```python
from build123d import *

# Parameters (mm, degrees)
CROQUIS1_W              = 128
CROQUIS1_H              = 98
SALIENTE_EXTRUIR1_DEPTH = 11.8
CROQUIS2_W              = 126
CROQUIS2_H              = 96
CORTAR_EXTRUIR1_DEPTH   = 11.3
SALIENTE_EXTRUIR2_DEPTH = 128
CROQUIS7_R              = 2.5
CORTAR_EXTRUIR2_DEPTH   = 22


with BuildPart() as part:
    # Croquis1 → Saliente-Extruir1 (new body)
    with BuildSketch(Plane.XY):
        with Locations((-9.684466696, -19.00455338)):
            Rectangle(CROQUIS1_W, CROQUIS1_H)
    extrude(amount=SALIENTE_EXTRUIR1_DEPTH)

    # Croquis2 → Cortar-Extruir1 (cut)
    with BuildSketch(Plane.XY.offset(11.8)):
        with Locations((-9.684466696, -19.00455338)):
            Rectangle(CROQUIS2_W, CROQUIS2_H)
    extrude(amount=-CORTAR_EXTRUIR1_DEPTH, mode=Mode.SUBTRACT)

    # Croquis5 → Saliente-Extruir2 (add)
    with BuildSketch(Plane.ZY.offset(73.684466696)):
        Polygon((0, -50.68455338), (-4.99696658, -47.79955338), (-4.99696658, 29.99544662), (0, 29.99544662), align=None)
    extrude(amount=-SALIENTE_EXTRUIR2_DEPTH)

    # Croquis7 → Cortar-Extruir2 (cut)
    with BuildSketch(Plane(origin=(0, 0, -4.99696658), x_dir=(-1, 0, 0), z_dir=(0, 0, -1))):
        with Locations(Location((-43.751056656, -37.767924802, 0), (0, 0, 90))):
            Circle(CROQUIS7_R)
    extrude(amount=-CORTAR_EXTRUIR2_DEPTH, mode=Mode.SUBTRACT)


solid = part.part
```
CAD build for the part. Positions are in the model's coordinates, mm. A direction names the side the tool comes from. Round coordinates to 2 decimals unless told otherwise and drop trailing zeros. Loops run counter-clockwise (first coordinate to the right, second up) from the corner with the lowest first, then second, coordinate; pieces in that order, holes last. Notation, with made-up numbers: M -29,4.5 L 10,4.5 A27 cw 10,24.5 Z; hole C 78,77.25 d9. An arc over 180 degrees is marked long. Return JSON: item names as keys, results as strings. Group by question number.
(1) Saw through at A-A, the plane z = 2.5. List the corners of the cut face in (x, y).
(2) Wall check: probe 1 along X at (y, z) = (18, 7.5); probe 2 along Y at (x, z) = (31.5, 3.25); probe 3 along Z at (x, y) = (36, -61). Give the ranges that are in metal, low to high. Write a range as [from, to].
(3) Drop flat-ended pins along their axis: P1, Ø3, axis at x = 43.75, y = -37.77, coming from the +Z side; P2, Ø12, axis at x = -11, y = -39.5, coming from the +Z side; P3, Ø14, axis at x = 2.5, y = -57, coming from the -Z side. Give the stop position or say it passes through.
(4) Mould opens along Y. For faces 4 (the flat face through (-11, 28.995, 6)), 5 (the flat face through (-73.684, -18, 4)), 6 (the cylindrical face through (41.533, -36.614, -2.287)), 7 (the flat face through (-11, 29.995, 3)) say: +Y half, -Y half, draft (parallel to the pull), parting line (faces both ways), or undercut.
(5) Saw through at C-C, the plane x = 17. List the corners of the cut face in (y, z).
(6) Saw through at D-D, the plane y = -61.5. List the corners of the cut face in (x, z), and give its area (3 significant figures).
(7) Tool access for faces 1 (the flat face through (54.316, -18, 4)), 2 (the flat face through (53.316, -20, 6)), 3 (the flat face through (-11, -59, 0)): list every direction of +Z, -Z, +X, -X, +Y, -Y with a clear straight run to the whole face (end or side of a thin tool).
(8) Saw through at B-B, the plane y = -38.5. List the corners of the cut face in (x, z).
Answer list:
{
 "1": {"outline": "M -73.68,-68 L 54.32,-68 L 54.32,30 L -73.68,30 Z; hole M -72.68,-67 L 53.32,-67 L 53.32,29 L -72.68,29 Z"},
 "2": {"probe 1": "[-73.68, -72.68], [53.32, 54.32]", "probe 2": "[-68, -67], [29, 30]", "probe 3": "[0, 0.5]"},
 "3": {"P1": "through", "P2": "z = 0.5", "P3": "z = -1.19"},
 "4": {"face 4": "undercut", "face 5": "draft", "face 6": "undercut", "face 7": "+Y half"},
 "5": {"outline": "M -68,0 L -50.68,0 L -47.8,-5 L 30,-5 L 30,11.8 L 29,11.8 L 29,0.5 L -67,0.5 L -67,11.8 L -68,11.8 Z"},
 "6": {"outline": "M -73.68,0 L 54.32,0 L 54.32,11.8 L 53.32,11.8 L 53.32,0.5 L -72.68,0.5 L -72.68,11.8 L -73.68,11.8 Z", "area": "86.6 mm2"},
 "7": {"face 1": "+Z, -Z, +X, +Y, -Y", "face 2": "+Z", "face 3": "-Z, +X, -X, -Y"},
 "8": {"outline": "M -73.68,-5 L 41.36,-5 L 41.36,0.5 L -72.68,0.5 L -72.68,11.8 L -73.68,11.8 Z; M 46.14,-5 L 54.32,-5 L 54.32,11.8 L 53.32,11.8 L 53.32,0.5 L 46.14,0.5 Z"}
}
